Autodesk Inventor part; units mm, degrees
ref_plane "YZ Plane" through (0, 0, 0) normal (1, 0, 0) x (0, 1, 0)
ref_plane "XZ Plane" through (0, 0, 0) normal (0, 1, 0) x (-1, 0, 0)
ref_plane "XY Plane" through (0, 0, 0) normal (0, 0, 1) x (1, 0, 0)
sketch "Sketch1" plane through (0, 0, 0) normal (0, 0, 1) x (1, 0, 0)
  line L0 (0, 0) -> (-15, 0)
  line L1 (-15, 0) -> (-15, 4)
  line L2 (-15, 4) -> (-11, 5.6)
  line L3 (-11, 5.6) -> (-11, 6.6)
  line L4 (-11, 6.6) -> (0, 6.6)
  line L5 (0, 6.6) -> (0, 0)
  dimension "d1" = 4
  dimension "d5" = 1
  dimension "d12" = 11
  dimension "d13" = 2.6
  dimension "d14" = 4
revolve "Revolution1" add sketch "Sketch1" angle 360 about axis through (0, 6.6, 0) along (0, -1, 0)
fillet "Fillet1" radius 0.5 1 edges at (15, 0, 0)
sketch "Sketch3" plane through (0, 0, 0) normal (0, -1, 0) x (1, 0, 0)
  circle A0 centre (0, 0) radius 2.5
  dimension "d15" = 5
extrude "Extrusion2" cut sketch "Sketch3" against normal up to surface (6.6 mm away)
fillet "Fillet2" radius 0.4 1 edges at (15, 4, 0)
sketch "Sketch4" plane through (0, 6.6, 0) normal (0, 1, 0) x (1, 0, 0)
  circle A0 centre (0, 0) radius 8
  circle A1 centre (0, 0) radius 6.1
  dimension "d19" = 16
  dimension "d20" = 1.9
extrude "Extrusion3" add sketch "Sketch4" along normal blind 1
properties part number "pulley"
Work out the finished part from the listing and answer in its coordinate system (mm). A direction names the side the tool comes from. Give positions to 0.01 mm unless a question says otherwise; leave off trailing zeros. Loops run counter-clockwise (first coordinate to the right, second up) from the corner with the lowest first, then second, coordinate; pieces in that order, holes last. Notation, with made-up numbers: (0.5, 79.5) -> (5.5, 79.5) arc R13 cw to (5.5, 88.5) -> close; hole circle Ø9 at (63.5, -24.75). An arc over 180 degrees is marked (long way). Use CSV: the item, a comma, the result in double quotes.
1. The part is cut by section A-A (y = 1). Write down the section's boundary in (x, z).
Found:
outline,"circle Ø30 at (0, 0); hole circle Ø5 at (0, 0)"
2. Flat-ended cylindrical pins translate along their axes: pin 1 Ø4 at (x, z) = (-11.5, -11.5) entering from +Y; pin 2 Ø1 at (y, z) = (2.5, 5.5) entering from -X; pin 3 Ø2 at (x, z) = (9.5, -2) entering from +Y. Find the tip coordinate at first contact, or state that the pin passes through.
Found:
pin 1,"y = 4.29"
pin 2,"x = -14.14"
pin 3,"y = 6.6"
3. The mould has two halves that part along Z. Classify faces 1 (the flat face through (-2, 7.6, 6)), 2 (the cylindrical face through (-6.094, 7.093, 0.268)), 3 (the cylindrical face through (-1.73, 7.09, -7.81)): +Z half, -Z half, draft (parallel to the pull), parting line (faces both ways), or undercut.
Found:
face 1,"draft"
face 2,"undercut"
face 3,"parting line"
4. A tool of negligible diameter and unlimited length cuts with its end or side. For faces 4 (the cylindrical face through (-0.54, 3.25, -2.44)), 5 (the cylindrical face through (2.38, 6.11, -10.74)), from which of +Z, -Z, +X, -X, +Y, -Y can it reach the whole face along a straight path? Write none if from no direction.
Found:
face 4,"+Y, -Y"
face 5,"+Y"
5. Straight lines are drawn through the part: line 1 (Z direction, x = 0, y = 3.25); line 2 (X direction, y = 7.1, z = 0). For each, find the intervals that lie inside material, in ascending order.
Found:
line 1,"-15 to -2.5, 2.5 to 15"
line 2,"-8 to -6.1, 6.1 to 8"
